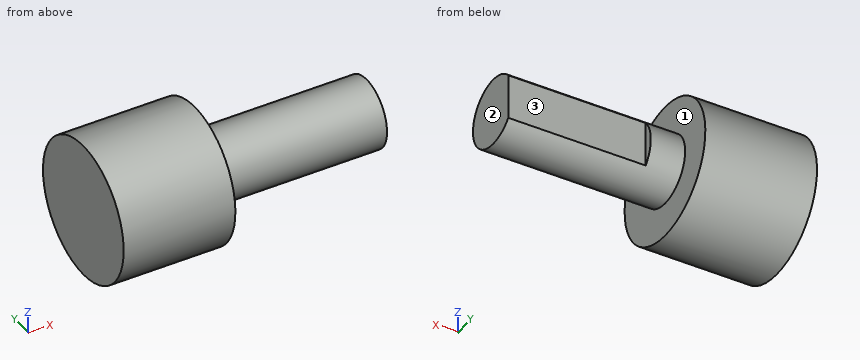
```python
from build123d import *

# Parameters (mm, degrees)
ESQUISSE1_R             = 4
BOSS_EXTRU_1_DEPTH      = 6.5
ESQUISSE2_R             = 2
BOSS_EXTRU_2_DEPTH      = 10
ESQUISSE3_W             = 4
ESQUISSE3_H             = 0.5
ENL_V_MAT_EXTRU_1_DEPTH = 8


with BuildPart() as part:
    # Esquisse1 → Boss.-Extru.1 (new body)
    with BuildSketch(Plane(origin=(0, 0, 0), x_dir=(0, 0, -1), z_dir=(1, 0, 0))):
        Circle(ESQUISSE1_R)
    extrude(amount=BOSS_EXTRU_1_DEPTH)

    # Esquisse2 → Boss.-Extru.2 (add)
    with BuildSketch(Plane(origin=(6.5, 0, 0), x_dir=(0, 0, -1), z_dir=(1, 0, 0))):
        Circle(ESQUISSE2_R)
    extrude(amount=BOSS_EXTRU_2_DEPTH)

    # Esquisse3 → Enlèv. mat.-Extru.1 (cut)
    with BuildSketch(Plane(origin=(16.5, 0, 0), x_dir=(0, 0, -1), z_dir=(1, 0, 0))):
        with Locations((0, 1.75)):
            Rectangle(ESQUISSE3_W, ESQUISSE3_H)
    extrude(amount=-ENL_V_MAT_EXTRU_1_DEPTH, mode=Mode.SUBTRACT)


solid = part.part
```
The listing builds one solid part. Answer for the finished solid, in the listing's coordinates (mm). Face numbers are marked on the shaded views. A direction names the side the tool comes from. Give positions to 0.01 mm unless a question says otherwise; leave off trailing zeros. Loops run counter-clockwise (first coordinate to the right, second up) from the corner with the lowest first, then second, coordinate; pieces in that order, holes last. Notation, with made-up numbers: (84, -7) - (109, -7) arc R30 ccw to (109, 31) - close; hole circle Ø1 at (76.5, 67.25). An arc over 180 degrees is marked (long way). Answer as CSV lines item,"result". Start each with the question number.
Item 1: For the marked faces 1, 2 and 3, determine the directions among +Z, -Z, +X, -X, +Y, -Y from which every point of the face is accessible in a straight line to the end or side of a thin tool.
Item 2: Each of these flat-tipped pins is pushed along its axis until it touches: pin 1 (1.5 mm diameter, centred on x = 9.5, z = 3, fed in from +Y); pin 2 (3 mm diameter, centred on x = 6, y = 2.5, fed in from -Z); pin 3 (2 mm diameter, centred on x = 11.5, z = 2.5, fed in from -Y); pin 4 (3 mm diameter, centred on x = 9, y = 2.5, fed in from -Z). Where does it stop, or does it pass through?
Item 3: A cutting plane is placed at A-A on y = 0. Determine the outline of the cut face in (x, z), then the cut area to 3 significant figures.
Item 4: A cutting plane is placed at C-C on x = 5.5. Determine the outline of the cut face in (y, z), then the cut area to 3 significant figures.
Item 5: A cutting plane is placed at D-D on y = -1. Determine the outline of the cut face in (x, z).
Item 6: Find the intervals of material crossed by line 1 (X direction, y = -1.5, z = -3); line 2 (Z direction, x = 11.5, y = -1.5), in increasing order. Write a range as from..to.
Item 7: A cutting plane is placed at B-B on z = 0. Determine the outline of the cut face in (x, y).
Found:
1,face 1,"+X"
1,face 2,"+Z, -Z, +X, +Y, -Y"
1,face 3,"+Z, -Z, +X, +Y"
2,pin 1,"passes through"
2,pin 2,"stops at z = -3.87"
2,pin 3,"stops at y = -1.32"
2,pin 4,"stops at z = -1.73"
3,outline,"(0, -4) - (6.5, -4) - (6.5, -2) - (16.5, -2) - (16.5, 2) - (6.5, 2) - (6.5, 4) - (0, 4) - close"
3,area,"92.0 mm^2"
4,outline,"circle Ø8 at (0, 0)"
4,area,"50.3 mm^2"
5,outline,"(0, -3.87) - (6.5, -3.87) - (6.5, -1.73) - (16.5, -1.73) - (16.5, 1.73) - (6.5, 1.73) - (6.5, 3.87) - (0, 3.87) - close"
6,line 1,"x = 0..6.5"
6,line 2,"z = -1.32..1.32"
7,outline,"(0, -4) - (6.5, -4) - (6.5, -2) - (16.5, -2) - (16.5, 1.5) - (8.5, 1.5) - (8.5, 2) - (6.5, 2) - (6.5, 4) - (0, 4) - close"
